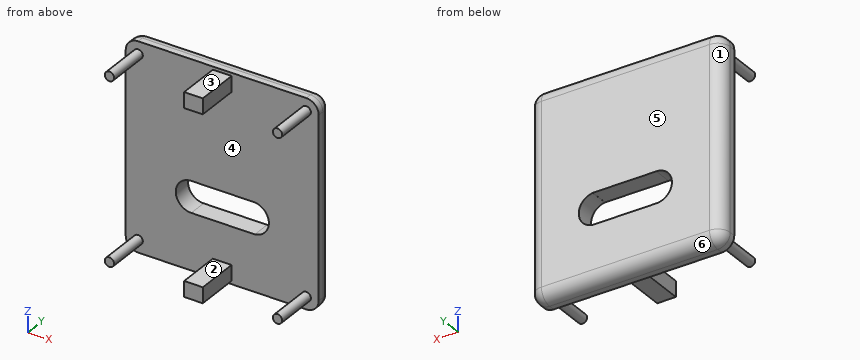
Autodesk Inventor part; units mm, degrees
ref_plane "YZ Plane" through (0, 0, 0) normal (1, 0, 0) x (0, 1, 0)
ref_plane "XZ Plane" through (0, 0, 0) normal (0, 1, 0) x (-1, 0, 0)
ref_plane "XY Plane" through (0, 0, 0) normal (0, 0, 1) x (1, 0, 0)
sketch "Boceto1" plane through (0, 0, 0) normal (0, 1, 0) x (-1, 0, 0)
  line L0 (15.5, 16.5) -> (-15.5, 16.5)
  line L1 (-15.5, 16.5) -> (-15.5, -16.5)
  line L2 (-15.5, -16.5) -> (15.5, -16.5)
  line L3 (15.5, -16.5) -> (15.5, 16.5)
  line L4 (-15.5, 16.5) -> (15.5, -16.5) construction
  circle A0 centre (15.5, -16.5) radius 0
  line L5 (0, -20.441182) -> (0, -13.180985)
  circle A1 centre (-15.5, -16.5) radius 0
  line L6 (0, 0) -> (-6.703667, 0)
  circle A2 centre (15.5, 16.5) radius 0
  circle A3 centre (-15.5, 16.5) radius 0
  line L7 (-1.743284, -16.5) -> (-1.743284, -13.5)
  line L8 (-1.743284, -13.5) -> (-1.743284, 1.5)
  line L9 (-1.743284, 1.5) -> (-1.743284, 3.5)
  line L10 (-1.743284, 3.5) -> (-1.743284, 13.5)
  line L11 (-1.743284, 13.5) -> (-1.743284, 16.5)
  line L12 (15.5, 0) -> (12.5, 0)
  line L13 (12.5, 0) -> (-12.5, 0)
  line L14 (-12.5, 0) -> (-15.5, 0)
  line L15 (-0.653653, 1.5) -> (-0.653653, -3.5)
  line L16 (12.5, 0) -> (12.5, -5)
  line L17 (12.5, -5) -> (2.466636, -5)
  line L18 (-15.5, 0) -> (-15.5, -5)
  line L19 (-15.5, -5) -> (-12.5, -5)
  circle A4 centre (4.966636, -5) radius 2.5
  line L20 (0, -8.467064) -> (0, -3.5)
  line L21 (12.5, -5) -> (7.5, -5)
  line L22 (12.5, -5) -> (-15.5, -5)
  line L23 (-12.5, -5) -> (-7.5, -5)
  line L24 (-7.5, -5.492671) -> (-7.5, -4.332105)
  line L25 (-7.5, -7.321441) -> (-7.5, -3.5)
  line L26 (-7.5, -5) -> (-3.010459, -5)
  line L27 (-5.25523, -5) -> (-5.25523, -7.5)
  line L28 (-5.25523, -7.5) -> (-3.485236, -7.5)
  line L29 (-5.25523, -5) -> (-5.25523, -2.5)
  line L30 (-5.25523, -2.5) -> (-3.924845, -2.5)
  circle A5 centre (-5, -5) radius 2.5
  line L31 (4.966636, -7.5) -> (-5.25523, -7.5)
  line L32 (-5.25523, -2.5) -> (4.966636, -2.5)
  point P0 (-5.25523, -2.513063)
  point P1 (-5.25523, -7.486937)
  dimension "d0" = 31
  dimension "d1" = 33
  dimension "d3" = 3
  dimension "d4" = 15
  dimension "d5" = 2
  dimension "d6" = 10
  dimension "d7" = 3
  dimension "d8" = 3
  dimension "d9" = 25
  dimension "d10" = 3
  dimension "d11" = 5
  dimension "d12" = 5
  dimension "d14" = 5
  dimension "d15" = 3
  dimension "d16" = 5
  dimension "d17" = 5
  dimension "d19" = 5
  dimension "d21" = 2.5
  dimension "d22" = 2.5
sketch "Boceto1 outline for Extrusión1" plane through (0, 0, 0) normal (0, 1, 0) x (-1, 0, 0)
  line L0 (-15.5, -16.5) -> (15.5, -16.5)
  line L1 (-15.5, 16.5) -> (-15.5, -16.5)
  line L2 (15.5, -16.5) -> (15.5, 16.5)
  line L3 (15.5, 16.5) -> (-15.5, 16.5)
  arc A0 (-5.25523, -7.486937) -> (-5.25523, -2.513063) centre (-5, -5) cw
  line L4 (-5.25523, -7.5) -> (-5.25523, -7.486937)
  line L5 (-3.485236, -7.5) -> (-5.25523, -7.5)
  line L6 (4.966636, -7.5) -> (-3.485236, -7.5)
  arc A1 (4.966636, -2.5) -> (4.966636, -7.5) centre (4.966636, -5) cw
  line L7 (-3.924845, -2.5) -> (4.966636, -2.5)
  line L8 (-5.25523, -2.5) -> (-3.924845, -2.5)
  line L9 (-5.25523, -2.513063) -> (-5.25523, -2.5)
extrude "Extrusión1" add sketch "Boceto1 outline for Extrusión1" along normal blind 3
fillet "Empalme1" radius 2 8 edges at (-15.5, 1.5, 16.5) (-15.5, 3, 0) (-15.5, 1.5, -16.5) (0, 3, -16.5) (15.5, 3, 0) (0, 3, 16.5) (15.5, 1.5, 16.5) (15.5, 1.5, -16.5)
sketch "Boceto2" plane through (0, 0, 0) normal (0, -1, 0) x (1, 0, 0)
  line L0 (-13.5, -14.5) -> (13.5, -14.5)
  circle A0 centre (13.5, -14.5) radius 0.75
  line L1 (0, -0.514663) -> (0, 1.763645)
  circle A1 centre (-13.5, -14.5) radius 0.75
  line L2 (0.998187, 0) -> (-3.186461, 0)
  circle A2 centre (13.5, 14.5) radius 0.75
  circle A3 centre (-13.5, 14.5) radius 0.75
  arc A4 (15.5, 14.5) -> (13.5, 16.5) centre (13.5, 14.5) ccw
  arc A5 (-13.5, 16.5) -> (-15.5, 14.5) centre (-13.5, 14.5) ccw
  arc A6 (-15.5, -14.5) -> (-13.5, -16.5) centre (-13.5, -14.5) ccw
  arc A7 (13.5, -16.5) -> (15.5, -14.5) centre (13.5, -14.5) ccw
  line L3 (-15.5, -14.5) -> (-15.5, 14.5)
  line L4 (-15.5, -14.5) -> (-1.5, -14.5)
  line L5 (-1.5, -14.5) -> (1, -14.5)
  line L6 (13.5, -14.5) -> (13.5, -13.5)
  line L7 (13.5, -14.5) -> (13.5, 14.5)
  line L8 (13.5, -13.5) -> (-13.5, -13.5)
  line L9 (-13.5, 14.5) -> (-13.5, -14.5)
  line L10 (15.5, 14.5) -> (15.5, -14.5)
  line L11 (15.5, -13.5) -> (1.5, -13.5)
  line L12 (-15.5, -13.5) -> (-1.5, -13.5)
  line L13 (1.5, -13.5) -> (1.5, -16)
  line L14 (1.5, -16) -> (-1.5, -16)
  line L15 (-1.5, -16) -> (-1.5, -13.5)
  line L16 (-1.5, 14.5) -> (1, 14.5)
  line L17 (1.5, 13.5) -> (1.5, 16)
  line L18 (1.5, 16) -> (-1.5, 16)
  line L19 (-1.5, 16) -> (-1.5, 13.5)
  line L20 (13.5, 14.5) -> (-13.5, 14.5)
  line L21 (0.770935, 14.5) -> (1.5, 14.5)
  line L22 (-1.5, 16) -> (-1.5, 13.5)
  line L23 (1.5, 13.5) -> (-1.5, 13.5)
  dimension "d26" = 1.5
  dimension "d27" = 14
  dimension "d28" = 2.5
  dimension "d29" = 1
  dimension "d30" = 14
  dimension "d31" = 14
  dimension "d32" = 2.5
extrude "Extrusión2" add sketch "Boceto2" along normal blind 7 contours L9 A1 L0 | L0 A1 L4 | L4 A1 L9 | L15 L8 L13 L0 | L0 L13 L14 L15 | L9 L20 A3 | A3 L20 L9 | A0 L6 L0 | L0 L6 A0 | L19 L18 L17 L20 L16 | L16 L20 L17 L23 L19 | L7 L20 A2 | A2 L20 L7
properties part number "TapaCajaNodoReceptor"
For this review, take the finished solid that the model builds, in its own axes (mm). Face numbers are marked on the shaded views. A direction names the side the tool comes from. Give positions to 0.01 mm unless a question says otherwise; leave off trailing zeros. Write each loop counter-clockwise with the first axis right and the second up, starting at its lowest first coordinate (ties: lowest second). Pieces come first, ordered by that corner, then holes.
Item 1: The part is to be moulded in two halves that separate along Z. For the marked faces 3, 4, 5 and 6, say which applies: +Z half, -Z half, draft (parallel to the pull), parting line (faces both ways), or undercut.
Item 2: Insertion check: P1, Ø5, axis at x = -1, z = 3.5, coming from the -Y side; P2, Ø1.2, axis at y = -4.5, z = 14, coming from the +X side; P3, Ø3, axis at y = -4.5, z = -14.5, coming from the -X side. Each pin has a flat end and moves straight along its axis. Give the tip position at first contact, or say it passes through.
Item 3: Wall thickness on probe 1 along Z at (x, y) = (0, -2); probe 2 along Y at (x, z) = (8.5, 11); probe 3 along Z at (x, y) = (-13, -6.25): over which ranges is each line inside the solid? List them lowest first.
Item 4: Take a section at B-B (y = -2.5). Give the boundary of the cut face in (x, z), and give its area (3 significant figures).
Item 5: Take a section at A-A (x = 6.5). Give the boundary of the cut face in (y, z).
Item 6: Machinability: for the marked faces 1 and 2, which of the approach directions +Z, -Z, +X, -X, +Y, -Y give a long, thin tool a straight path to every point of the face, cutting with its end or side? Answer none if there is none.
Item 7: Take a section at C-C (z = -5). Give the boundary of the cut face in (x, y).
Established:
1. face 3: +Z half
1. face 4: undercut
1. face 5: draft
1. face 6: -Z half
2. P1: stops at y = 0
2. P2: stops at x = 14.25
2. P3: stops at x = -14.25
3. probe 1: z = -16 to -13.5, 13.5 to 16
3. probe 2: y = 0 to 3
3. probe 3: z = -15.06 to -13.94, 13.94 to 15.06
4. outline: circle Ø1.5 at (-13.5, -14.5); circle Ø1.5 at (-13.5, 14.5); (-1.5, -16) - (1.5, -16) - (1.5, -13.5) - (-1.5, -13.5) - close; (-1.5, 13.5) - (1.5, 13.5) - (1.5, 16) - (-1.5, 16) - close; circle Ø1.5 at (13.5, -14.5); circle Ø1.5 at (13.5, 14.5)
4. area: 22.1 mm2
5. outline: (0, -16.5) - (1, -16.5) arc R2 ccw to (3, -14.5) - (3, -7) - (0, -7) - close; (0, -3) - (3, -3) - (3, 14.5) arc R2 ccw to (1, 16.5) - (0, 16.5) - close
6. face 1: +Z, -Z, -X, +Y
6. face 2: +X, -X, -Y
7. outline: (-15.5, 0) - (-7.47, 0) - (-7.47, 3) - (-13.5, 3) arc R2 ccw to (-15.5, 1) - close; (7.5, 0) - (15.5, 0) - (15.5, 1) arc R2 ccw to (13.5, 3) - (7.5, 3) - close
